Read the model definition and answer for the solid it produces. Units are mm, in the model's axes. Face numbers are marked on the shaded views. A direction names the side the tool comes from. Give positions to 0.01 mm unless a question says otherwise; leave off trailing zeros. Order: outer loops, then holes, each group sorted by start corner. A loop starts at its lowest first (then second) coordinate and runs counter-clockwise, first axis right, second up. Notation, with made-up numbers: (40.5, -38.5) -> (52.5, -38.5) arc R25 cw to (52.5, -23.5) -> close; hole circle Ø8 at (79, 25). An arc over 180 degrees is marked (long way). Use one line per item in the form item = value.
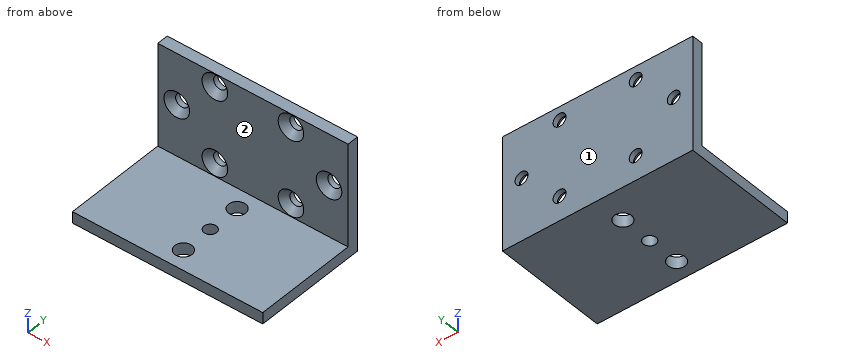
```python
from build123d import *

# Parameters (mm, degrees)
F0_W           = 50
F0_H           = 27
F1_DEPTH       = 3
F2_D           = 3.4
F2_CSINK_D     = 6.72
F2_CSINK_ANGLE = 90
F3_DEPTH       = 3
F0_H_2         = 3
F4_DEPTH       = 27
F6_D           = 3.3
F7_D           = 4.5


with BuildPart() as f1:
    # F0 (on Front) → F1 (new body)
    with BuildSketch(Plane.XZ):
        with Locations((25, 16.5)):
            Rectangle(F0_W, F0_H)
    extrude(amount=-F1_DEPTH)

    # F2 (through all)
    with Locations(Plane.XZ):
        with Locations((35, 26.5), (15, 26.5), (15, 6.5), (35, 6.5), (5, 16.5), (45, 16.5)):
            CounterSinkHole(F2_D / 2, F2_CSINK_D / 2, counter_sink_angle=F2_CSINK_ANGLE)

    # F3 (add): a face of the model
    f3_faces = [f1.faces().sort_by_distance(p)[0] for p in [
        (25, 1.5, 3),
    ]]
    extrude(f3_faces, amount=F3_DEPTH)

    # F0 (on Front) → F4 (join)
    with BuildSketch(Plane.XZ):
        with Locations((25, 1.5)):
            Rectangle(F0_W, F0_H_2)
    extrude(amount=F4_DEPTH)

    # F6 (through all)
    with Locations(Plane.XY.offset(3)):
        with Locations((25, -13.5)):
            Hole(F6_D / 2)

    # F7 (through all)
    with Locations(Plane.XY.offset(3)):
        with Locations((25, -5), (25, -22)):
            Hole(F7_D / 2)


solid = f1.part
```
Item 1: Straight lines are drawn through the part: L1, parallel to X at y = 2, z = 6.5; L2, parallel to X at y = 2.5, z = 16.5; L3, parallel to Z at x = 35, y = 2.05. For each, find the intervals that lie inside material, in ascending order. Write a range as from..to.
Checks:
L1 = 0..13.3, 16.7..33.3, 36.7..50
L2 = 0..3.3, 6.7..43.3, 46.7..50
L3 = 0..4.8, 8.2..24.8, 28.2..30
Item 2: Which of the six approach directions +Z, -Z, +X, -X, +Y, -Y give full straight-line access (tool end or side, diameter ignored) to the marked faces 1 and 2?
Checks:
face_1 = +Z, -Z, +X, -X, +Y
face_2 = +Z, +X, -X, -Y
Item 3: The part is cut by section B-B on y = -13.5. Give the vertices of the cut face in (x, z).
Checks:
outline = (0, 0) -> (23.35, 0) -> (23.35, 3) -> (0, 3) -> close; (26.65, 0) -> (50, 0) -> (50, 3) -> (26.65, 3) -> close
Item 4: Given pin 1 Ø4.5 at (x, z) = (35, 26.5) entering from -Y; pin 2 Ø13.5 at (x, z) = (37.5, 11) entering from -Y; pin 3 Ø5.5 at (x, z) = (5, 16.5) entering from -Y, each flat-ended and moving along its own axis, determine where each tip first touches the part or whether it passes through.
Checks:
pin_1 = 1.11
pin_2 = 0
pin_3 = 0.61
Item 5: The part is cut by section C-C on z = 6.5. Give the vertices of the cut face in (x, y), and give its area (3 significant figures).
Checks:
outline = (0, 0) -> (11.64, 0) -> (13.3, 1.66) -> (13.3, 3) -> (0, 3) -> close; (16.7, 1.66) -> (18.36, 0) -> (31.64, 0) -> (33.3, 1.66) -> (33.3, 3) -> (16.7, 3) -> close; (36.7, 1.66) -> (38.36, 0) -> (50, 0) -> (50, 3) -> (36.7, 3) -> close
area = 124 mm²
Item 6: The part is cut by section A-A on x = 15. Give the vertices of the cut face in (y, z), and give its area (3 significant figures).
Checks:
outline = (-27, 0) -> (3, 0) -> (3, 4.8) -> (1.66, 4.8) -> (0, 3.14) -> (0, 3) -> (-27, 3) -> close; (0, 9.86) -> (1.66, 8.2) -> (3, 8.2) -> (3, 24.8) -> (1.66, 24.8) -> (0, 23.14) -> close; (0, 29.86) -> (1.66, 28.2) -> (3, 28.2) -> (3, 30) -> (0, 30) -> close
area = 145 mm²
Item 7: The part is cut by section D-D on x = 5. Give the vertices of the cut face in (y, z).
Checks:
outline = (-27, 0) -> (3, 0) -> (3, 14.8) -> (1.66, 14.8) -> (0, 13.14) -> (0, 3) -> (-27, 3) -> close; (0, 19.86) -> (1.66, 18.2) -> (3, 18.2) -> (3, 30) -> (0, 30) -> close
